Geometry: final body of the model. Coordinates: model frame, mm. Coordinates: 2 decimals unless noted, no trailing zeros. Write each loop counter-clockwise with the first axis right and the second up, starting at its lowest first coordinate (ties: lowest second). Pieces come first, ordered by that corner, then holes. Notation, with made-up numbers: (59.25, -13.75) - (79.25, -13.75) arc R19 cw to (79.25, 2.25) - close; hole circle Ø4 at (44.5, -38). An arc over 180 degrees is marked (long way). Answer as a JSON object with one key per item and string values. Group by question number.
Item 1: Section A-A on z = 13.5. Return loops of the section in (x, y), and give its area (3 significant figures).
Item 2: Section D-D on x = 0. Return loops of the section in (y, z), and give its area (3 significant figures).
Item 3: Line query: line 1 along X through (y, z) = (7.5, 12); line 2 along Z through (x, y) = (-0.5, 14); line 3 along Z through (x, y) = (-5.5, 13.5). Output: solid intervals per line, ascending. Write a range as from..to.
Item 4: Section C-C on x = 16. Return loops of the section in (y, z).
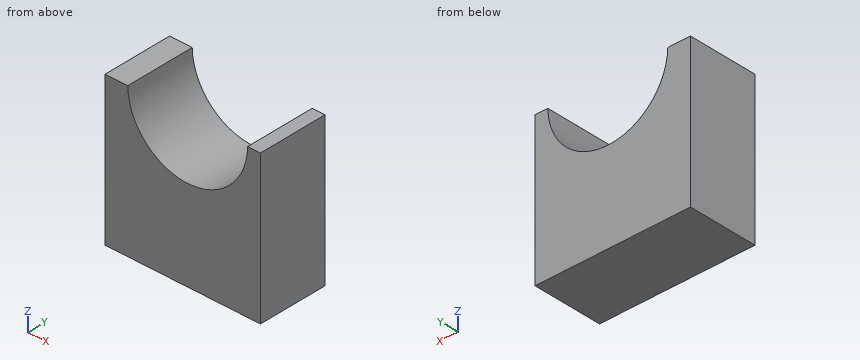
```python
from build123d import *

# Parameters (mm, degrees)
F0_W     = 77.63347
F0_H     = 66.146884
F1_DEPTH = 30.734
F2_R     = 26.443213
F3_DEPTH = 31.496
F5_DEPTH = 78.486
F6_DEPTH = 70.358


with BuildPart() as f1:
    # F0 (on Front) → F1 (new body)
    with BuildSketch(Plane.XZ):
        with Locations((2.376534, 0.792177)):
            Rectangle(F0_W, F0_H)
    extrude(amount=-F1_DEPTH)

    # F2 (on Front) → F3 (cut)
    with BuildSketch(Plane.XZ):
        with Locations((0, 34.261707)):
            Circle(F2_R)
    extrude(amount=-F3_DEPTH, mode=Mode.SUBTRACT)

    # F4 (on Top) → F5 (cut)
    with BuildSketch(Plane.XY):
        Polygon((32.083217, 39.410867), (32.083217, 31.092994), (32.083217, 0), (41.589357, 0), (41.589357, 39.410867), align=None)
    extrude(amount=F5_DEPTH, mode=Mode.SUBTRACT)

    # F4 (on Top) → F6 (cut)
    with BuildSketch(Plane.XY):
        Polygon((32.083217, 39.410867), (32.083217, 31.092994), (32.083217, 0), (41.589357, 0), (41.589357, 39.410867), align=None)
    extrude(amount=-F6_DEPTH, mode=Mode.SUBTRACT)


solid = f1.part
```
Checks:
{
 "1": {"outline": "(-36.44, 0) - (-16.38, 0) - (-16.38, 30.73) - (-36.44, 30.73) - close; (16.38, 0) - (32.08, 0) - (32.08, 30.73) - (16.38, 30.73) - close", "area": "1,100 mm^2"},
 "2": {"outline": "(0, -32.28) - (30.73, -32.28) - (30.73, 7.82) - (0, 7.82) - close", "area": "1,230 mm^2"},
 "3": {"line 1": "-36.44..-14.27, 14.27..32.08", "line 2": "-32.28..7.82", "line 3": "-32.28..8.4"},
 "4": {"outline": "(0, -32.28) - (30.73, -32.28) - (30.73, 13.21) - (0, 13.21) - close"}
}
